Verification items for the finished model (mm, model axes). A direction names the side the tool comes from. Give positions to 0.01 mm unless a question says otherwise; leave off trailing zeros. Loops run counter-clockwise (first coordinate to the right, second up) from the corner with the lowest first, then second, coordinate; pieces in that order, holes last. Notation, with made-up numbers: M -18,-14 L -3,-14 A23 cw -3,7 Z; hole C -17,-8 d5. An arc over 180 degrees is marked long. Use CSV: the item, a comma, the result in double quotes.
Autodesk Inventor part; units mm, degrees
ref_plane "YZ Plane" through (0, 0, 0) normal (1, 0, 0) x (0, 1, 0)
ref_plane "XZ Plane" through (0, 0, 0) normal (0, 1, 0) x (-1, 0, 0)
ref_plane "XY Plane" through (0, 0, 0) normal (0, 0, 1) x (1, 0, 0)
sketch "Sketch1" plane through (0, 0, 0) normal (0, 0, 1) x (1, 0, 0)
  circle A0 centre (0, 0) radius 63.5
  line L0 (0, 0) -> (0, 63.5) construction
  line L1 (-6.35, 76.2) -> (6.35, 76.2)
  line L2 (6.35, 76.2) -> (6.35, 0)
  line L3 (6.35, 0) -> (-6.35, 0) construction
  line L4 (-6.35, 0) -> (-6.35, 76.2)
  line L5 (-6.35, 76.2) -> (6.35, 0) construction
  line L6 (6.35, 76.2) -> (-6.35, 0) construction
  circle A1 centre (0, 0) radius 50.8
  circle A2 centre (0, 0) radius 19.05
  line L7 (-69.1661, -32.6007) -> (-3.175, 5.4993)
  line L8 (3.175, -5.4993) -> (-62.8161, -43.5993)
  line L9 (62.8161, -43.5993) -> (-3.175, -5.4993)
  line L10 (3.175, 5.4993) -> (69.1661, -32.6007)
  circle A3 centre (0, 0) radius 12.7 construction
  circle A4 centre (6.35, 10.9985) radius 1.7526
  line L11 (0, 0) -> (6.35, 10.9985) construction
  circle A5 centre (-6.35, 10.9985) radius 1.7526
  circle A6 centre (-12.7, 0) radius 1.7526
  circle A7 centre (-6.35, -10.9985) radius 1.7526
  circle A8 centre (6.35, -10.9985) radius 1.7526
  circle A9 centre (12.7, 0) radius 1.7526
  circle A10 centre (0, 0) radius 7.9375
  circle A11 centre (0, 57.15) radius 3.175
  arc A12 (-40.474, -30.7) -> (40.474, -30.7) centre (0, 13.0686) ccw
  point P0 (0, 38.1)
  point P1 (-6.35, 50.4016)
  point P2 (-6.35, 17.9605)
  point P3 (-18.7293, -3.481)
  point P4 (-46.824, -19.7015)
  point P5 (-6.35, 63.1817)
  point P6 (6.35, 63.1817)
  point P7 (-12.3793, -14.4795)
  point P8 (12.3793, -14.4795)
  point P9 (40.474, -30.7)
  point P10 (6.35, 50.4016)
  point P11 (46.824, -19.7015)
  point P12 (18.7293, -3.481)
  point P13 (6.35, 17.9605)
  point P14 (0, -46.5455)
  dimension "d0" = 127
  dimension "d9" = 25.4
  dimension "d1" = 76.2
  dimension "d2" = 12.7
  dimension "d3" = 12.7
  dimension "d4" = 38.1
  dimension "d7" = 360
  dimension "d10" = 3.5052
  dimension "d11" = 30
  dimension "d14" = 360
  dimension "d16" = 15.875
  dimension "d17" = 6.35
  dimension "d18" = 57.15
  dimension "d22" = 46.5455
extrude "Extrusion1" add sketch "Sketch1" along normal blind 6.35 contours A0 L10 A1 L2 | L2 A1 L4 A0 | A0 L4 L1 L2 | A0 L9 A1 L10 | L4 A1 L7 A0 | L2 A2 L4 A1 | A0 L8 A1 L9 | A1 L9 A2 L10 | L7 A1 L8 A0 | A2 L10 A9 A10 L2 A4 | L2 A4 A10 L4 A5 A2 | A1 A12 | A2 L9 A8 A10 L10 A9 | L7 A2 L8 A1 | L4 A5 A10 L7 A6 A2 | A2 L8 A7 A10 L9 A8 | L7 A6 A10 L8 A7 A2 | A11
fillet "Fillet1" radius 3.175 14 edges at (6.35, 50.4016, 3.175) (6.35, 17.9605, 3.175) (18.7293, -3.481, 3.175) (46.824, -19.7015, 3.175) (12.3793, -14.4795, 3.175) (-12.3793, -14.4795, 3.175) (-18.7293, -3.481, 3.175) (-6.35, 17.9605, 3.175) (-46.824, -19.7015, 3.175) (-6.35, 50.4016, 3.175) (-6.35, 63.1817, 3.175) (6.35, 63.1817, 3.175) (40.474, -30.7, 3.175) (-40.474, -30.7, 3.175)
properties part number "Emma Blade"
(1) Section check B-B on y = -26. Record the cut outline in (x, z), plus the area to 3 significant figures.
Calculated:
outline,"M -57.93,0 L -32.33,0 L -32.33,6.35 L -57.93,6.35 Z; M 32.33,0 L 57.93,0 L 57.93,6.35 L 32.33,6.35 Z"
area,"325 mm²"
(2) Section check C-C on x = -29.5. Record the cut outline in (y, z).
Calculated:
outline,"M -56.23,0 L -38.73,0 L -38.73,6.35 L -56.23,6.35 Z; M -24.36,0 L -9.7,0 L -9.7,6.35 L -24.36,6.35 Z; M 41.36,0 L 56.23,0 L 56.23,6.35 L 41.36,6.35 Z"
(3) Tool access check on faces 5 (the flat face through (-0.9, -8.2, 6.35)), 6 (the flat face through (-6.35, 71, 3)), 7 (the cylindrical face through (-46.336, -18.037, 3.219)). Record the directions out of +Z, -Z, +X, -X, +Y, -Y that give a thin tool (end or side, any length) a straight path to the whole face; none if there is none.
Calculated:
face 5,"+Z, +X, -X, +Y, -Y"
face 6,"+Z, -Z, -X, +Y"
face 7,"+Z, -Z"
(4) Mould release check, pull along Y, two halves, no side actions. Record for faces 1 (the cylindrical face through (-7.146, 63.889, 3.219)), 2 (the flat face through (-6.35, 33, 3)), 3 (the cylindrical face through (2.665, -63.444, 3.131)), 4 (the flat face through (6.35, 71, 3)): released by +Y, released by -Y, zero draft, split by the parting line, or undercut.
Calculated:
face 1,"released by +Y"
face 2,"undercut"
face 3,"split by the parting line"
face 4,"zero draft"
(5) Section check A-A on x = 0. Record the cut outline in (y, z), plus the area to 3 significant figures.
Calculated:
outline,"M -63.5,0 L -46.55,0 L -46.55,6.35 L -63.5,6.35 Z; M -19.05,0 L -7.94,0 L -7.94,6.35 L -19.05,6.35 Z; M 7.94,0 L 76.2,0 L 76.2,6.35 L 7.94,6.35 Z"
area,"612 mm²"
(6) Depth check by flat-ended pin: pin 1 Ø1 at (x, z) = (50.5, 4) entering from +Y; pin 2 Ø3 at (x, z) = (-7, 2) entering from -Y. Enter the tip coordinate at first touch or a pass-through.
Calculated:
pin 1,"stops at y = 39.14"
pin 2,"stops at y = -63.26"
(7) Section check D-D on z = 5. Count the separate pieces of the cut face and the enclosed holes in it, plus the area to 3 significant figures.
Calculated:
separate pieces,"1"
enclosed holes,"10"
area,"7,110 mm²"
(8) Scan lines: L1, parallel to X at y = 0, z = 5; L2, parallel to Y at x = 0, z = 3.5; L3, parallel to X at y = 43.5, z = 2. Record each from-to range of solid material in increasing order. Write a range as from..to.
Calculated:
L1,"x = -63.5..-50.8, -19.05..-14.45, -10.95..-7.94, 7.94..10.95, 14.45..19.05, 50.8..63.5"
L2,"y = -63.5..-46.55, -19.05..-7.94, 7.94..76.2"
L3,"x = -46.26..-26.24, -6.35..6.35, 26.24..46.26"
